Drawing for the job (mm, zero at the part's lowest x, y, z). Coordinates: 2 decimals unless noted, no trailing zeros. Write each loop counter-clockwise with the first axis right and the second up, starting at its lowest first coordinate (ties: lowest second). Pieces come first, ordered by that corner, then holes. Notation, with made-up numbers: M 25,56.5 L 82,56.5 A34 cw 82,86.5 Z; hole C 86.5,32 d4. An arc over 180 degrees is marked long. Put each result on its own line as item: value. Start each with the question number.
Q1. Cut at C-C (x = 15). Write the cut outline in (y, z).
Q2. Drop flat-ended pins along their axis: pin 1 (0.9 mm diameter, centred on y = 2, z = 2, fed in from +X); pin 2 (0.9 mm diameter, centred on y = 2, z = 35, fed in from -X); pin 3 (0.9 mm diameter, centred on y = 1, z = 17.5, fed in from -X). Give the stop position or say it passes through.
Q3. Cut at B-B (z = 18). Write the cut outline in (x, y), then the cut area to 3 significant figures.
Q4. Drill centre lines: line 1 along X through (y, z) = (0.4, 2.5); line 2 along Z through (x, y) = (2, 0.7); line 3 along X through (y, z) = (1.55, 34.5). Where is each one in solid material? Low to high.
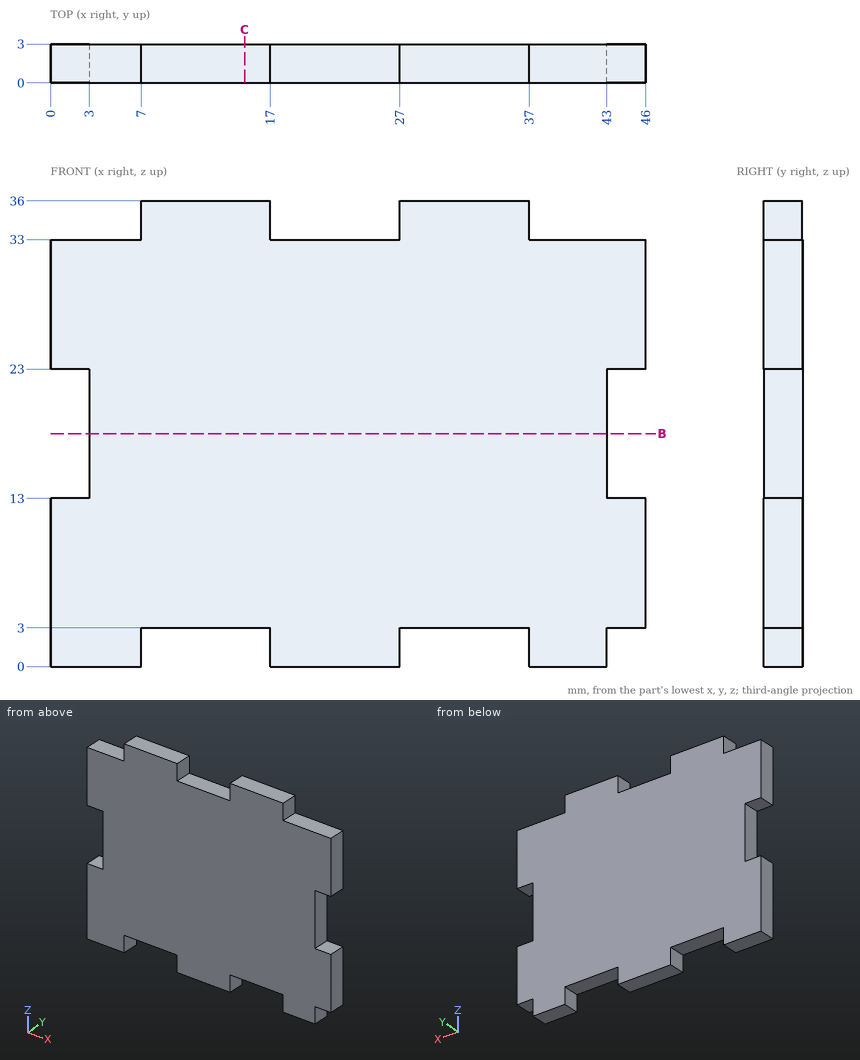
Computed values:
1. outline: M 0,3 L 3,3 L 3,36 L 0,36 Z
2. pin 1: x = 43
2. pin 2: x = 7
2. pin 3: x = 3
3. outline: M 3,0 L 43,0 L 43,3 L 3,3 Z
3. area: 120 mm2
4. line 1: 0 to 7, 17 to 27, 37 to 43
4. line 2: 0 to 13, 23 to 33
4. line 3: 7 to 17, 27 to 37
